CAD build for the part. Positions are in the model's coordinates, mm. A direction names the side the tool comes from. Coordinates: 2 decimals unless noted, no trailing zeros. Write each loop counter-clockwise with the first axis right and the second up, starting at its lowest first coordinate (ties: lowest second). Pieces come first, ordered by that corner, then holes. Notation, with made-up numbers: (-14, 62.25) - (37, 62.25) arc R28 cw to (37, 101.25) - close; hole circle Ø9 at (33, 9). An arc over 180 degrees is marked (long way). One line per question, with ' | ' between items. Start each with the question number.
1. Which spindle directions (+Z, -Z, +X, -X, +Y, -Y) get a long thin tool onto all of the face, cutting with end or side? Do faces 1 (the flat face through (0, 1.1, 2)), 2 (the flat face through (0, -1.1, 2)), 3 (the flat face through (0, 6.9, -1)). Say none if no direction does.
2. Flat gauge pins, fed straight in: P1, Ø2.5, axis at x = 0, z = 2, coming from the -Y side; P2, Ø1, axis at x = 1, z = 1.5, coming from the +Y side; P3, Ø2, axis at x = -1, y = 5.5, coming from the +Z side. Where does each tip first touch, or does it go through?
3. Probe line 1 (Z direction, x = 2.5, y = 4); line 2 (Y direction, x = 5, z = 4.75); line 3 (X direction, y = -0.5, z = 1.5). List the from-to ranges inside material, lowest first.
4. Band-saw the part on B-B, the plane y = 0. Write the cut outline in (x, z), then the cut area to 3 significant figures.
5. Band-saw the part on D-D, the plane y = 3.75. Write the cut outline in (x, z).
6. Band-saw the part on C-C, the plane x = -6.5. Write the cut outline in (y, z), then the cut area to 3 significant figures.
7. Band-saw the part on A-A, the plane x = -3. Write the cut outline in (y, z).
from build123d import *

# Parameters (mm, degrees)
F0_W     = 12.1
F0_H     = 2.2
F1_DEPTH = 5
F0_W_2   = 15
F0_H_2   = 9
F2_DEPTH = 1.5
F3_R     = 0.75


with BuildPart() as f1:
    # F0 (on Top) → F1 (new body)
    with BuildSketch(Plane.XY):
        Rectangle(F0_W, F0_H)
    extrude(amount=F1_DEPTH)

    # F0 (on Top) → F2 (join)
    with BuildSketch(Plane.XY):
        with Locations((0, 2.4)):
            Rectangle(F0_W_2, F0_H_2)
        Rectangle(F0_W, F0_H, mode=Mode.SUBTRACT)
        Rectangle(F0_W, F0_H)
    extrude(amount=-F2_DEPTH)

    # F3
    f3_edges = [f1.edges().sort_by_distance(p)[0] for p in [
        (-6.05, 1.1, 2.5),
        (-6.05, -1.1, 2.5),
        (6.05, 1.1, 2.5),
        (6.05, -1.1, 2.5),
        (7.5, -2.1, -0.75),
        (7.5, 6.9, -0.75),
        (-7.5, 6.9, -0.75),
        (-7.5, -2.1, -0.75),
    ]]
    fillet(f3_edges, radius=F3_R)


solid = f1.part
Filled in:
1) face 1: +Z, +X, -X, +Y | face 2: +Z, +X, -X, -Y | face 3: +Z, -Z, +X, -X, +Y
2) P1: stops at y = -1.1 | P2: stops at y = 1.1 | P3: stops at z = 0
3) line 1: z = -1.5 to 0 | line 2: y = -1.1 to 1.1 | line 3: x = -6.03 to 6.03
4) outline: (-7.5, -1.5) - (7.5, -1.5) - (7.5, 0) - (6.05, 0) - (6.05, 5) - (-6.05, 5) - (-6.05, 0) - (-7.5, 0) - close | area: 83.0 mm²
5) outline: (-7.5, -1.5) - (7.5, -1.5) - (7.5, 0) - (-7.5, 0) - close
6) outline: (-2.1, -1.5) - (6.9, -1.5) - (6.9, 0) - (-2.1, 0) - close | area: 13.5 mm²
7) outline: (-2.1, -1.5) - (6.9, -1.5) - (6.9, 0) - (1.1, 0) - (1.1, 5) - (-1.1, 5) - (-1.1, 0) - (-2.1, 0) - close
